Autodesk Inventor part; units mm, degrees
ref_plane "YZ Plane" through (0, 0, 0) normal (1, 0, 0) x (0, 1, 0)
ref_plane "XZ Plane" through (0, 0, 0) normal (0, 1, 0) x (-1, 0, 0)
ref_plane "XY Plane" through (0, 0, 0) normal (0, 0, 1) x (1, 0, 0)
sketch "Sketch1" plane through (0, 0, 0) normal (0, 1, 0) x (-1, 0, 0)
  line L0 (3.8, 16.8) -> (-3.8, 16.8)
  line L1 (-3.8, 16.8) -> (-3.8, -16.8)
  line L2 (-3.8, -16.8) -> (3.8, -16.8)
  line L3 (3.8, -16.8) -> (3.8, 16.8)
  circle A0 centre (0, 14.15) radius 1.6
  circle A1 centre (0, -14.15) radius 1.6
  point P0 (0, 0)
  dimension "d0" = 33.6
  dimension "d1" = 7.6
  dimension "d2" = 16.8
  dimension "d3" = 3.8
  dimension "d4" = 3.2
  dimension "d5" = 3.2
  dimension "d6" = 28.3
  dimension "d7" = 14.15
extrude "Extrusion1" add sketch "Sketch1" along normal blind 2.4
fillet "Fillet1" radius 1 4 edges at (3.8, 1.2, 16.8) (-3.8, 1.2, 16.8) (3.8, 1.2, -16.8) (-3.8, 1.2, -16.8)
sketch "Sketch2" plane through (0, 2.4, 0) normal (0, 1, 0) x (1, 0, 0)
  line L0 (-3.05, -9.6694) -> (-3.05, 9.6694)
  line L1 (-3.05, 9.6694) -> (3.05, 11.9)
  line L2 (3.05, 11.9) -> (3.05, -11.9)
  line L3 (3.05, -11.9) -> (-3.05, -9.6694)
  line L4 (2.55, -11.1848) -> (-2.55, -9.3198)
  line L5 (-2.55, -9.3198) -> (-2.55, 9.3198)
  line L6 (-2.55, 9.3198) -> (2.55, 11.1848)
  line L7 (2.55, 11.1848) -> (2.55, -11.1848)
  point P0 (0, 0)
  dimension "d11" = 69.914
  dimension "d13" = 23.8
  dimension "d14" = 6.1
  dimension "d15" = 3.05
  dimension "d17" = 0.5
  dimension "d18" = 0.5
  dimension "d19" = 0.5
  dimension "d20" = 0.5
  dimension "d21" = 11.9
  dimension "d22" = 69.914
  dimension "d23" = 69.914
extrude "Extrusion2" add sketch "Sketch2" along normal blind 4.6
fillet "Fillet2" radius 1 8 edges at (-3.05, 4.7, -9.6694) (-3.05, 4.7, 9.6694) (3.05, 4.7, 11.9) (3.05, 4.7, -11.9) (-2.55, 4.7, -9.3198) (-2.55, 4.7, 9.3198) (2.55, 4.7, -11.1848) (2.55, 4.7, 11.1848)
sketch "Sketch3" plane through (0, 0, 0) normal (0, -1, 0) x (1, 0, 0)
  line L0 (3.4, 12) -> (-3.4, 12)
  line L1 (-3.4, 12) -> (-3.4, -12)
  line L2 (-3.4, -12) -> (3.4, -12)
  line L3 (3.4, -12) -> (3.4, 12)
  point P0 (0, 0)
  dimension "d27" = 24
  dimension "d28" = 6.8
  dimension "d29" = 12
  dimension "d30" = 3.4
extrude "Extrusion3" add sketch "Sketch3" along normal blind 3.5
equation "\"d5\" = d4"
equation "\"d22\" = d11"
properties part number "31pin female connector"
Design review of the part built by this model. Coordinates are the model's own, in mm. A direction names the side the tool comes from. Coordinates: 2 decimals unless noted, no trailing zeros. Order: outer loops, then holes, each group sorted by start corner. A loop starts at its lowest first (then second) coordinate and runs counter-clockwise, first axis right, second up.
Item 1: The part is to be moulded in two halves that separate along X. For faces 5 (the flat face through (-2.55, 5, 0)), 6 (the flat face through (-3.4, -2, 0)), 7 (the flat face through (-3.3, 2.4, 0.2)), say which applies: pulls with the +X half, pulls with the -X half, needs draft (parallel to the pull), parting line crosses it, or undercut.
Item 2: For pin 1 Ø2.5 at (x, z) = (0, 2.5) entering from +Y; pin 2 Ø1.9 at (x, z) = (0, 14.15) entering from +Y; pin 3 Ø1.8 at (x, y) = (1, -1.5) entering from +Z; pin 4 Ø5 at (y, z) = (5, -2.5) entering from -X, all flat-tipped, find the tip position at first contact; note any pin that passes through.
Item 3: For faces 1 (the cylindrical face through (-2.365, 4.732, -9.201)), 2 (the cylindrical face through (-2.9, 4.7, 9.5)), 3 (the cylindrical face through (2.61, 4.73, 11.3)), 4 (the flat face through (0, -2, 12)), list the 3-axis set-ups (+Z, -Z, +X, -X, +Y, -Y) from which the entire face can be reached by the end or side of a thin tool; tool diameter is ignored.
Item 4: For line 1 (Z direction, x = 0, y = 1.95); line 2 (X direction, y = 5.5, z = 9); line 3 (Z direction, x = 1, y = 3.5), list the stretches that pass through material, from the lowest coordinate up.
Item 5: Take a section at D-D, the plane z = -1. Write out the cut boundary in (x, y), then the cut area to 3 significant figures.
Item 6: Take a section at C-C, the plane x = 0.75. Write out the cut boundary in (y, z).
Item 7: Take a section at A-A, the plane y = 3. Write out the cut boundary in (x, z).
Item 8: Take a section at B-B, the plane z = 14.15. Write out the cut boundary in (x, y).
The answers:
1. face 5: undercut
1. face 6: pulls with the -X half
1. face 7: needs draft
2. pin 1: stops at y = 2.4
2. pin 2: passes through
2. pin 3: stops at z = 12
2. pin 4: stops at x = -3.05
3. face 1: +Y
3. face 2: +Z, -X, +Y
3. face 3: +Z, +Y
3. face 4: +Z, +X, -X, -Y
4. line 1: z = -16.8 to -15.75, -12.55 to 12.55, 15.75 to 16.8
4. line 2: x = -3.05 to -2.48, 2.55 to 3.05
4. line 3: z = -11.15 to -10.62, 10.62 to 11.15
5. outline: (-3.8, 0) - (-3.4, 0) - (-3.4, -3.5) - (3.4, -3.5) - (3.4, 0) - (3.8, 0) - (3.8, 2.4) - (3.05, 2.4) - (3.05, 7) - (2.55, 7) - (2.55, 2.4) - (-2.55, 2.4) - (-2.55, 7) - (-3.05, 7) - (-3.05, 2.4) - (-3.8, 2.4) - close
5. area: 46.6 mm2
6. outline: (-3.5, -12) - (0, -12) - (0, -12.74) - (2.4, -12.74) - (2.4, -11.06) - (7, -11.06) - (7, -10.53) - (2.4, -10.53) - (2.4, 10.53) - (7, 10.53) - (7, 11.06) - (2.4, 11.06) - (2.4, 12.74) - (0, 12.74) - (0, 12) - (-3.5, 12) - close; (0, -16.8) - (2.4, -16.8) - (2.4, -15.56) - (0, -15.56) - close; (0, 15.56) - (2.4, 15.56) - (2.4, 16.8) - (0, 16.8) - close
7. outline: (-3.05, -8.97) arc R1 ccw to (-2.39, -9.91) - (1.71, -11.41) arc R1 ccw to (3.05, -10.47) - (3.05, 10.47) arc R1 ccw to (1.71, 11.41) - (-2.39, 9.91) arc R1 ccw to (-3.05, 8.97) - close; hole (-2.55, -8.62) arc R1 ccw to (-1.89, -9.56) - (1.21, -10.69) arc R1 ccw to (2.55, -9.75) - (2.55, 9.75) arc R1 ccw to (1.21, 10.69) - (-1.89, 9.56) arc R1 ccw to (-2.55, 8.62) - close
8. outline: (-3.8, 0) - (-1.6, 0) - (-1.6, 2.4) - (-3.8, 2.4) - close; (1.6, 0) - (3.8, 0) - (3.8, 2.4) - (1.6, 2.4) - close
